from build123d import *

# Parameters (mm, degrees)
SKETCH1_W           = 110.49
SKETCH1_H           = 44.45
SKETCH1_W_2         = 25.4
SKETCH1_H_2         = 25.4
BOSS_EXTRUDE1_DEPTH = 8.255
FILLET1_R           = 6.35
SKETCH2_R           = 4.445
BOSS_EXTRUDE2_DEPTH = 22.225
BOSS_EXTRUDE3_START = 22.225
SKETCH3_R           = 4.445
BOSS_EXTRUDE3_DEPTH = 22.225


with BuildPart() as part:
    # Sketch1 → Boss-Extrude1 (new, symmetric)
    with BuildSketch(Plane(origin=(0, 0, 0), x_dir=(1, 0, 0), z_dir=(0, 1, 0))):
        Rectangle(SKETCH1_W, SKETCH1_H)
        Rectangle(SKETCH1_W_2, SKETCH1_H_2, mode=Mode.SUBTRACT)
    extrude(amount=BOSS_EXTRUDE1_DEPTH, both=True)

    # Fillet1
    fillet1_edges = [part.edges().sort_by_distance(p)[0] for p in [
        (-55.245, 8.255, 0),
        (55.245, 8.255, 0),
        (-55.245, -8.255, 0),
        (55.245, -8.255, 0),
    ]]
    fillet(fillet1_edges, radius=FILLET1_R)

    # Sketch2 → Boss-Extrude2 (add)
    with BuildSketch(Plane.XY.offset(22.225)):
        with Locations(Location((-33.866666667, 0, 0), (0, 0, 180))):
            Circle(SKETCH2_R)
        with Locations(Location((33.866666667, 0, 0), (0, 0, 180))):
            Circle(SKETCH2_R)
    extrude(amount=BOSS_EXTRUDE2_DEPTH)

    # Sketch3 → Boss-Extrude3 (add)
    with BuildSketch(Plane(origin=(0, 0, -22.225), x_dir=(-1, 0, 0), z_dir=(0, 0, -1)).offset(BOSS_EXTRUDE3_START)):
        with Locations((-33.866666667, 0)):
            Circle(SKETCH3_R)
        with Locations((33.866666667, 0)):
            Circle(SKETCH3_R)
    extrude(amount=-BOSS_EXTRUDE3_DEPTH)


solid = part.part
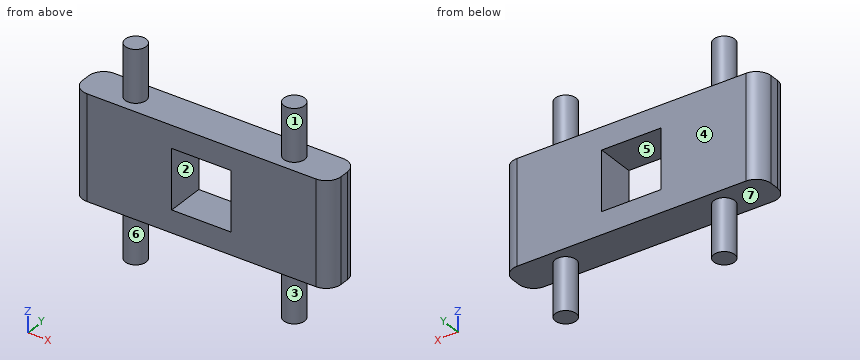
Input: part model. Units: mm. Frame: model coordinates. Face numbers are marked on the shaded views. A direction names the side the tool comes from. Give positions to 0.01 mm unless a question says otherwise; leave off trailing zeros. Loops run counter-clockwise (first coordinate to the right, second up) from the corner with the lowest first, then second, coordinate; pieces in that order, holes last. Notation, with made-up numbers: (-37, 31.5) - (17, 31.5) arc R19 ccw to (17, 62.5) - close; hole circle Ø4 at (33.25, -24.75). An arc over 180 degrees is marked (long way). Use CSV: the item, a comma, the result in double quotes. Start each with the question number.
Item 1: Section C-C on z = -15. Return loops of the section in (x, y) (3 decimals).
Item 2: Section D-D on x = 17.5. Return loops of the section in (y, z) (3 decimals), then the cut area to 3 significant figures.
Item 3: Reachability of the marked faces 1, 2, 3 and 4 from +Z, -Z, +X, -X, +Y, -Y: full face, straight path, thin tool, end or side. Return the list, or none.
Item 4: Mould query, pull axis Z, two halves, no side actions, for the marked faces 5, 6 and 7. Classes: pulls with the +Z half, pulls with the -Z half, needs draft (parallel to the pull), parting line crosses it, or undercut.
Item 5: Contact query for flat-ended pins moving along their axis: P1, Ø5, axis at x = 5, y = 2.5, coming from the -Z side (3 decimals); P2, Ø3, axis at x = 0, y = -1, coming from the +Z side (3 decimals); P3, Ø5, axis at y = -3, z = -26, coming from the -X side. Output: stop coordinate, or through.
Item 6: Section A-A on z = 1. Return loops of the section in (x, y) (3 decimals), then the cut area to 3 significant figures.
Item 7: Line query: line 1 (X direction, y = 2, z = 5); line 2 (Z direction, x = -11, y = -2.5) (3 decimals); line 3 (Z direction, x = -21, y = 4) (3 decimals). Output: solid intervals per line, ascending.
Item 8: Section B-B on y = 0. Return loops of the section in (x, z) (3 decimals).
Ans:
1,outline,"(-55.245, -1.905) arc R6.35 ccw to (-48.895, -8.255) - (48.895, -8.255) arc R6.35 ccw to (55.245, -1.905) - (55.245, 1.905) arc R6.35 ccw to (48.895, 8.255) - (-48.895, 8.255) arc R6.35 ccw to (-55.245, 1.905) - close"
2,outline,"(-8.255, -22.225) - (8.255, -22.225) - (8.255, 22.225) - (-8.255, 22.225) - close"
2,area,"734 mm2"
3,face 1,"+Z"
3,face 2,"+Y, -Y"
3,face 3,"-Z"
3,face 4,"+Z, -Z, +X, -X, +Y"
4,face 5,"undercut"
4,face 6,"needs draft"
4,face 7,"pulls with the -Z half"
5,P1,"stops at z = -22.225"
5,P2,"stops at z = 22.225"
5,P3,"stops at x = -38.28"
6,outline,"(-55.245, -1.905) arc R6.35 ccw to (-48.895, -8.255) - (-12.7, -8.255) - (-12.7, 8.255) - (-48.895, 8.255) arc R6.35 ccw to (-55.245, 1.905) - close; (12.7, -8.255) - (48.895, -8.255) arc R6.35 ccw to (55.245, -1.905) - (55.245, 1.905) arc R6.35 ccw to (48.895, 8.255) - (12.7, 8.255) - close"
6,area,"1,370 mm2"
7,line 1,"x = -55.24 to -12.7, 12.7 to 55.24"
7,line 2,"z = -22.225 to -12.7, 12.7 to 22.225"
7,line 3,"z = -22.225 to 22.225"
8,outline,"(-55.245, -22.225) - (-38.312, -22.225) - (-38.312, -44.45) - (-29.422, -44.45) - (-29.422, -22.225) - (29.422, -22.225) - (29.422, -44.45) - (38.312, -44.45) - (38.312, -22.225) - (55.245, -22.225) - (55.245, 22.225) - (38.312, 22.225) - (38.312, 44.45) - (29.422, 44.45) - (29.422, 22.225) - (-29.422, 22.225) - (-29.422, 44.45) - (-38.312, 44.45) - (-38.312, 22.225) - (-55.245, 22.225) - close; hole (-12.7, -12.7) - (12.7, -12.7) - (12.7, 12.7) - (-12.7, 12.7) - close"
